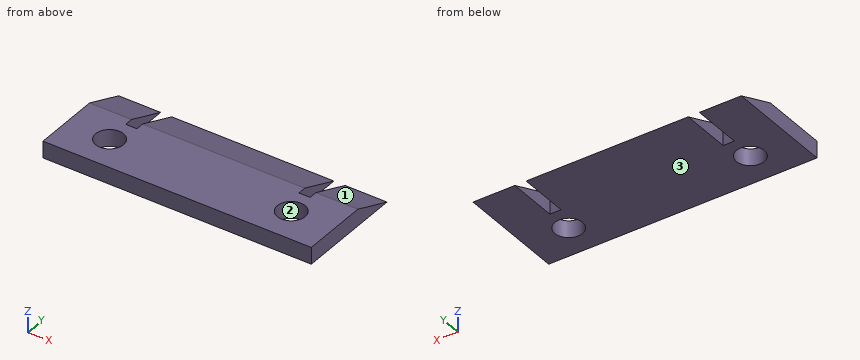
from build123d import *

# Parameters (mm, degrees)
SKETCH_1_W               = 96
SKETCH_1_H               = 39
EXTRUDE_1_DEPTH          = 6
CUT_EXTRUDE_1_DEPTH      = 104.793063352
CUT_EXTRUDE_1_DEPTH_BACK = 104.793063352
SKETCH_3_W               = 4
SKETCH_3_H               = 18
CUT_EXTRUDE_1_2_DEPTH    = 63.136945532
SKETCH_4_R               = 5
CUT_EXTRUDE_2_DEPTH      = 63.136945532


with BuildPart() as part:
    # 草图1 → 凸台-拉伸1 (new body)
    with BuildSketch(Plane.XY):
        with Locations((0, 19.5)):
            Rectangle(SKETCH_1_W, SKETCH_1_H)
    extrude(amount=EXTRUDE_1_DEPTH)

    # 草图2 → Cut-Extrude 1 (cut, two sides: drawn at the far end of the back side and taken through both)
    with BuildSketch(Plane(origin=(48, 0, 0), x_dir=(0, 0, -1), z_dir=(1, 0, 0)).offset(-CUT_EXTRUDE_1_DEPTH_BACK)):
        Polygon((-39.023196805, -58.557992014), (-6, 24), (0, 39), (33.023196805, 121.557992014), (-132.092787222, 187.604385624), (-204.139180832, 7.488401597), align=None)
    extrude(amount=CUT_EXTRUDE_1_DEPTH + CUT_EXTRUDE_1_DEPTH_BACK, mode=Mode.SUBTRACT)

    # 草图3 → Cut-Extrude 1 2 (cut, symmetric)
    with BuildSketch(Plane.XY.offset(6)):
        with Locations((-31, 30)):
            Rectangle(SKETCH_3_W, SKETCH_3_H)
    cut_extrude_1_2 = extrude(amount=CUT_EXTRUDE_1_2_DEPTH, both=True, mode=Mode.SUBTRACT)

    # 镜向1: Cut-Extrude 1 2 across plane
    add(cut_extrude_1_2.mirror(Plane(origin=(0, 0, 0), x_dir=(0, 0, 1), z_dir=(1, 0, 0))), mode=Mode.SUBTRACT)

    # 草图4 → 切除-拉伸2 (cut, through all)
    with BuildSketch(Plane.XY.offset(6)):
        with Locations((32.5, 12)):
            Circle(SKETCH_4_R)
        with Locations((-32.5, 12)):
            Circle(SKETCH_4_R)
    extrude(amount=-CUT_EXTRUDE_2_DEPTH, mode=Mode.SUBTRACT)


solid = part.part
The listing builds one solid part. Answer for the finished solid, in the listing's coordinates (mm). Face numbers are marked on the shaded views. Coordinates: 2 decimals unless noted, no trailing zeros. Write each loop counter-clockwise with the first axis right and the second up, starting at its lowest first coordinate (ties: lowest second). Pieces come first, ordered by that corner, then holes. Notation, with made-up numbers: M -25.5,-18 L 6.5,-18 A5 cw 6.5,-13 Z; hole C -38,7.5 d5. An arc over 180 degrees is marked long. Write each question's results on one line, items separated by ' | '.
Item 1: For a pull along Y with two mould halves and no side action, classify the marked faces 1, 2 and 3 as released by +Y, released by -Y, zero draft, split by the parting line, or undercut.
Answer below:
face 1: released by +Y | face 2: undercut | face 3: zero draft
Item 2: Consider probe 1 along X at (y, z) = (30.5, 2.5); probe 2 along Y at (x, z) = (32.5, 4.3); probe 3 along X at (y, z) = (15, 1.75). Determine where each line is inside the solid, lowest interval first. Write a range as [from, to].
Answer below:
probe 1: [-48, -33], [-29, 29], [33, 48] | probe 2: [0, 7], [17, 21] | probe 3: [-48, -36.5], [-28.5, 28.5], [36.5, 48]
Item 3: The part is cut by section B-B on z = 1.5. Determine the outline of the cut face in (x, y).
Answer below:
outline: M -48,0 L 48,0 L 48,35.25 L 33,35.25 L 33,21 L 29,21 L 29,35.25 L -29,35.25 L -29,21 L -33,21 L -33,35.25 L -48,35.25 Z; hole C -32.5,12 d10; hole C 32.5,12 d10
Item 4: The part is cut by section D-D on y = 32. Determine the outline of the cut face in (x, z).
Answer below:
outline: M -48,0 L -33,0 L -33,2.8 L -48,2.8 Z; M -29,0 L 29,0 L 29,2.8 L -29,2.8 Z; M 33,0 L 48,0 L 48,2.8 L 33,2.8 Z
Item 5: The part is cut by section A-A on y = 27.5. Determine the outline of the cut face in (x, z), and give its area (3 significant figures).
Answer below:
outline: M -48,0 L -33,0 L -33,4.6 L -48,4.6 Z; M -29,0 L 29,0 L 29,4.6 L -29,4.6 Z; M 33,0 L 48,0 L 48,4.6 L 33,4.6 Z | area: 405 mm2
Item 6: Given P1, Ø8, axis at x = -32.5, y = 12, coming from the -Z side; P2, Ø2, axis at x = 23.5, z = 5, coming from the +Y side, each flat-ended and moving along its own axis, determine where each tip first touches the part or whether it passes through.
Answer below:
P1: through | P2: y = 29
Item 7: The part is cut by section C-C on x = -31. Determine the outline of the cut face in (y, z).
Answer below:
outline: M 0,0 L 7.23,0 L 7.23,6 L 0,6 Z; M 16.77,0 L 21,0 L 21,6 L 16.77,6 Z
